Read the model definition and answer for the solid it produces. Units are mm, in the model's axes. Face numbers are marked on the shaded views. A direction names the side the tool comes from. Coordinates: 2 decimals unless noted, no trailing zeros. Loops run counter-clockwise (first coordinate to the right, second up) from the corner with the lowest first, then second, coordinate; pieces in that order, holes last.
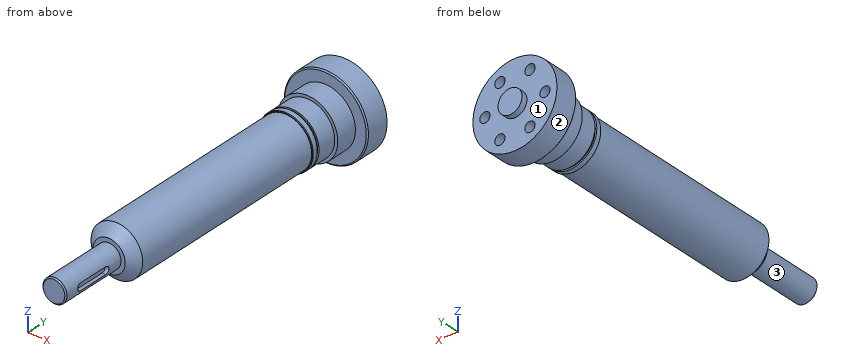
from build123d import *

# Parameters (mm, degrees)
F0_R      = 10
F1_DEPTH  = 56
F2_R      = 21.5
F3_DEPTH  = 180
F4_SIZE   = 8
F6_R      = 22.5
F7_DEPTH  = 40.35
F8_R      = 35
F9_DEPTH  = 20
F11_R     = 31.0096244967
F11_R_2   = 21.25
F12_DEPTH = 1.85
F15_DEPTH = 25
F16_SIZE  = 1
F18_SIZE  = 0.5
F17_R     = 10
F19_DEPTH = 5
F22_D     = 8.5
F22_DEPTH = 17
F22_TIP   = 2.5536576309
F23_SIZE  = 1
F25_R     = 25
F26_DEPTH = 18


with BuildPart() as f1:
    # F0 (on Front) → F1 (new body)
    with BuildSketch(Plane.XZ):
        Circle(F0_R)
    extrude(amount=F1_DEPTH)

    # F2 (on Front) → F3 (join)
    with BuildSketch(Plane.XZ):
        Circle(F2_R)
    extrude(amount=-F3_DEPTH)

    # F4
    f4_edges = [f1.edges().sort_by_distance(p)[0] for p in [
        (-21.5, 0, 0),
    ]]
    chamfer(f4_edges, length=F4_SIZE)

    # F6 (on offset) → F7 (join)
    with BuildSketch(Plane(origin=(0, 180, 0), x_dir=(-1, 0, 0), z_dir=(0, 1, 0))):
        Circle(F6_R)
    extrude(amount=F7_DEPTH)

    # F8 (on face) → F9 (join)
    with BuildSketch(Plane(origin=(0, 220.35, 0), x_dir=(-1, 0, 0), z_dir=(0, 1, 0))):
        Circle(F8_R)
    extrude(amount=F9_DEPTH)

    # F11 (on offset) → F12 (cut)
    with BuildSketch(Plane(origin=(0, 184.5, 0), x_dir=(-1, 0, 0), z_dir=(0, 1, 0))):
        Circle(F11_R)
        Circle(F11_R_2, mode=Mode.SUBTRACT)
    extrude(amount=F12_DEPTH, mode=Mode.SUBTRACT)

    # F14 (on offset) → F15 (cut)
    with BuildSketch(Plane.YZ.offset(6.5)):
        with BuildLine():
            Line((-15, 2.8761793831), (-41, 2.8761793831))
            ThreePointArc((-41, 2.8761793831), (-44, -0.1238206169), (-41, -3.1238206169))
            Line((-41, -3.1238206169), (-15, -3.1238206169))
            ThreePointArc((-15, -3.1238206169), (-12, -0.1238206169), (-15, 2.8761793831))
        make_face()
    extrude(amount=F15_DEPTH, mode=Mode.SUBTRACT)

    # F16
    f16_edges = [f1.edges().sort_by_distance(p)[0] for p in [
        (-10, -56, 0),
    ]]
    chamfer(f16_edges, length=F16_SIZE)

    # F18
    f18_edges = [f1.edges().sort_by_distance(p)[0] for p in [
        (22.5, 180, 0),
    ]]
    chamfer(f18_edges, length=F18_SIZE)

    # F17 (on face) → F19 (join)
    with BuildSketch(Plane(origin=(0, 240.35, 0), x_dir=(-1, 0, 0), z_dir=(0, 1, 0))):
        Circle(F17_R)
    extrude(amount=F19_DEPTH)

    # F22
    with Locations(Plane(origin=(0, 240.35, 0), x_dir=(-1, 0, 0), z_dir=(0, 1, 0))):
        with Locations((-12.5, 21.6506350946), (12.5, 21.6506350946), (25, 0), (12.5, -21.6506350946), (-12.5, -21.6506350946), (-25, 0)):
            Hole(F22_D / 2, depth=F22_DEPTH)
            with Locations((0, 0, -(F22_DEPTH + F22_TIP / 2))):  # 118° drill point
                Cone(0, F22_D / 2, F22_TIP, mode=Mode.SUBTRACT)

    # F23
    f23_edges = [f1.edges().sort_by_distance(p)[0] for p in [
        (35, 220.35, 0),
    ]]
    chamfer(f23_edges, length=F23_SIZE)

    # F25 (on offset) → F26 (join)
    with BuildSketch(Plane.XZ.offset(-202.35)):
        Circle(F25_R)
    extrude(amount=-F26_DEPTH)


solid = f1.part
Item 1: A cutting plane is placed at A-A on y = 156.5. Determine the outline of the cut face in (x, z), then the cut area to 3 significant figures.
Numbers:
outline: circle Ø43 at (0, 0)
area: 1,450 mm2
Item 2: Given pin 1 (4 mm diameter, centred on x = 7.5, y = -5, fed in from -Z); pin 2 (1.5 mm diameter, centred on x = -10.5, z = 6.5, fed in from +Y); pin 3 (8 mm diameter, centred on y = 100, z = 4, fed in from +X), each flat-ended and moving along its own axis, determine where each tip first touches the part or whether it passes through.
Numbers:
pin 1: stops at z = -8.35
pin 2: stops at y = 240.35
pin 3: stops at x = 21.5
Item 3: Find the intervals of material crossed by line 1 along Z through (x, y) = (12, 227); line 2 along Y through (x, z) = (-17, -19); line 3 along X through (y, z) = (12, -1), in increasing order.
Numbers:
line 1: z = -32.88 to -25.87, -17.43 to 17.43, 25.87 to 32.88
line 2: y = 220.35 to 240.35
line 3: x = -21.48 to 21.48
Item 4: Which of the six approach directions +Z, -Z, +X, -X, +Y, -Y give full straight-line access (tool end or side, diameter ignored) to the marked faces 1, 2 and 3?
Numbers:
face 1: +Y
face 2: +Y, -Y
face 3: -Y
